```python
from build123d import *

# Parameters (mm, degrees)
EXTRUDE_1_DEPTH     = 235
SKETCH_3_R          = 1.5
CUT_EXTRUDE_1_DEPTH = 10
SKETCH_4_W          = 151
SKETCH_4_H          = 3
CUT_EXTRUDE_2_DEPTH = 5


with BuildPart() as part:
    # Эскиз1 → Бобышка-Вытянуть1 (new body)
    with BuildSketch(Plane(origin=(0, 0, 0), x_dir=(0, 0, -1), z_dir=(1, 0, 0))):
        Polygon((0, 0), (-10, 0), (-10, 3), (-3, 3), (-3, 10), (0, 10), align=None)
    extrude(amount=EXTRUDE_1_DEPTH)

    # Эскиз3 → Вырез-Вытянуть1 (cut)
    with BuildSketch(Plane(origin=(0, 3, 0), x_dir=(1, 0, 0), z_dir=(0, 1, 0))):
        with Locations((7.5, -6.5)):
            Circle(SKETCH_3_R)
        with Locations((227.5, -6.5)):
            Circle(SKETCH_3_R)
    extrude(amount=-CUT_EXTRUDE_1_DEPTH, mode=Mode.SUBTRACT)

    # Эскиз4 → Вырез-Вытянуть2 (cut)
    with BuildSketch(Plane.XY.offset(10)):
        with Locations((117.5, 1.5)):
            Rectangle(SKETCH_4_W, SKETCH_4_H)
    extrude(amount=-CUT_EXTRUDE_2_DEPTH, mode=Mode.SUBTRACT)


solid = part.part
```
Geometry check sheet. Reference: the model listing, model coordinates, mm. A direction names the side the tool comes from. Round coordinates to 2 decimals unless told otherwise and drop trailing zeros. Order: outer loops, then holes, each group sorted by start corner. A loop starts at its lowest first (then second) coordinate and runs counter-clockwise, first axis right, second up. Notation, with made-up numbers: (30.25, 87.5) - (64.25, 87.5) arc R14 ccw to (64.25, 92.5) - close; hole circle Ø9 at (-34, 17). An arc over 180 degrees is marked (long way). Use a Markdown table: item, result. Add a question column.
(1) Material ranges on line 1 along X through (y, z) = (1.45, 6.5); line 2 along Z through (x, y) = (227.5, 2.25); line 3 along Y through (x, z) = (215, 8.5), recorded low to high. Write a range as [from, to].
(2) Sectioned sample at B-B, the plane x = 179.5. Enter the section's corners in (y, z), and give its area (3 significant figures).
(3) Sectioned sample at C-C, the plane y = 7.75. Enter the section's corners in (x, z).
(4) Sectioned sample at D-D, the plane x = 27.5. Enter the section's corners in (y, z).
(5) Depth check by flat-ended pin: pin 1 (0.9 mm diameter, centred on x = 121, y = 1, fed in from +Z); pin 2 (1.5 mm diameter, centred on x = 51.5, y = 6.5, fed in from +Z). Enter the tip coordinate at first touch or a pass-through.
(6) Tool access check on faces 1 (the flat face through (116, 3, 4)), 2 (the flat face through (116, 5, 0)). Record the directions out of +Z, -Z, +X, -X, +Y, -Y that give a thin tool (end or side, any length) a straight path to the whole face; none if there is none.
(7) Sectioned sample at A-A, the plane z = 6.5. Enter the section's corners in (x, y), and give its area (3 significant figures).
Answers below:
| question | item | result |
|---|---|---|
| 1 | line 1 | [0, 6], [9, 42], [193, 226], [229, 235] |
| 1 | line 2 | [0, 5], [8, 10] |
| 1 | line 3 | [0, 3] |
| 2 | outline | (0, 0) - (10, 0) - (10, 3) - (3, 3) - (3, 5) - (0, 5) - close |
| 2 | area | 36.0 mm² |
| 3 | outline | (0, 0) - (235, 0) - (235, 3) - (0, 3) - close |
| 4 | outline | (0, 0) - (10, 0) - (10, 3) - (3, 3) - (3, 10) - (0, 10) - close |
| 5 | pin 1 | z = 5 |
| 5 | pin 2 | z = 3 |
| 6 | face 1 | +Z, +X, -X, +Y |
| 6 | face 2 | -Z, +X, -X, +Y, -Y |
| 7 | outline | (0, 0) - (6, 0) - (6, 3) - (0, 3) - close; (9, 0) - (42, 0) - (42, 3) - (9, 3) - close; (193, 0) - (226, 0) - (226, 3) - (193, 3) - close; (229, 0) - (235, 0) - (235, 3) - (229, 3) - close |
| 7 | area | 234 mm² |
